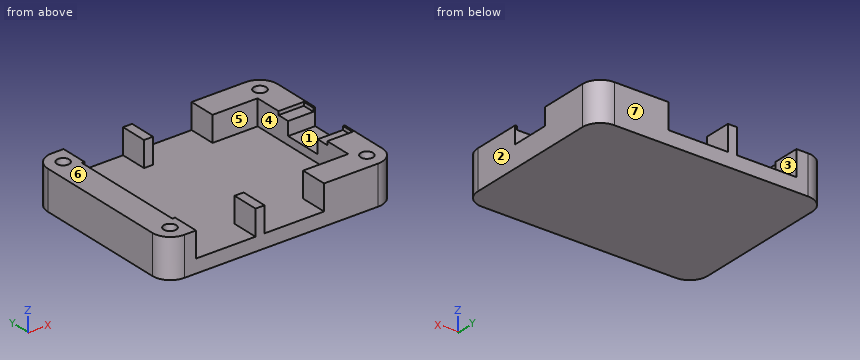
```python
from build123d import *

# Parameters (mm, degrees)
F0_R     = 2.6
F0_W     = 13.2
F0_H     = 6
F0_W_2   = 5.6
F0_H_2   = 8.5
F0_R_2   = 1.55
F0_H_3   = 2.75
F0_W_3   = 2
F0_R_3   = 1.375
F0_W_4   = 0.4
F1_DEPTH = 3
F2_DEPTH = 8.6
F3_DEPTH = 7.8
F4_DEPTH = 4.8


with BuildPart() as f1:
    # F0 (on Top) → F1 (new body)
    with BuildSketch(Plane.XY):
        Polygon((19.5, 13), (9.5, 13), (-3.7, 13), (-5.7, 13), (-18.9, 13), (-19.5, 13), (-19.5, -13), (-18.9, -13), (-5.7, -13), (-3.7, -13), (9.5, -13), (19.5, -13), (19.5, -7), (19.5, -4.25), (19.5, 4.25), (19.5, 7), align=None)
        with BuildLine():
            Line((-18.9, 13), (-18.9, 19))
            Line((-18.9, 19), (-21.5, 19))
            ThreePointArc((-21.5, 19), (-24.3284271247, 17.8284271247), (-25.5, 15))
            Line((-25.5, 15), (-25.5, -15))
            ThreePointArc((-25.5, -15), (-24.3284271247, -17.8284271247), (-21.5, -19))
            Line((-21.5, -19), (-18.9, -19))
            Line((-18.9, -19), (-18.9, -13))
            Line((-18.9, -13), (-19.5, -13))
            Line((-19.5, -13), (-19.5, 13))
            Line((-19.5, 13), (-18.9, 13))
        make_face()
        with Locations((-21.8334523779, -15.3334523779)):
            Circle(F0_R, mode=Mode.SUBTRACT)
        with Locations((-21.8334523779, 15.3334523779)):
            Circle(F0_R, mode=Mode.SUBTRACT)
        with BuildLine():
            Line((25.5, -15), (25.5, -7))
            Line((25.5, -7), (25.1, -7))
            Line((25.1, -7), (19.5, -7))
            Line((19.5, -7), (19.5, -13))
            Line((19.5, -13), (9.5, -13))
            Line((9.5, -13), (9.5, -19))
            Line((9.5, -19), (21.5, -19))
            ThreePointArc((21.5, -19), (24.3284271247, -17.8284271247), (25.5, -15))
        make_face()
        with Locations((21.8334523779, -15.3334523779)):
            Circle(F0_R, mode=Mode.SUBTRACT)
        with BuildLine():
            ThreePointArc((25.5, 15), (24.3284271247, 17.8284271247), (21.5, 19))
            Line((21.5, 19), (9.5, 19))
            Line((9.5, 19), (9.5, 13))
            Line((9.5, 13), (19.5, 13))
            Line((19.5, 13), (19.5, 7))
            Line((19.5, 7), (25.1, 7))
            Line((25.1, 7), (25.5, 7))
            Line((25.5, 7), (25.5, 15))
        make_face()
        with Locations((21.8334523779, 15.3334523779)):
            Circle(F0_R, mode=Mode.SUBTRACT)
        with Locations((-12.3, -16)):
            Rectangle(F0_W, F0_H)
        with Locations((2.9, 16)):
            Rectangle(F0_W, F0_H)
        with Locations((-12.3, 16)):
            Rectangle(F0_W, F0_H)
        with Locations((2.9, -16)):
            Rectangle(F0_W, F0_H)
        with Locations((22.3, 0)):
            Rectangle(F0_W_2, F0_H_2)
        with Locations((-21.8334523779, -15.3334523779)):
            Circle(F0_R)
        with Locations((-21.8334523779, -15.3334523779)):
            Circle(F0_R_2, mode=Mode.SUBTRACT)
        with Locations((21.8334523779, 15.3334523779)):
            Circle(F0_R)
        with Locations((21.8334523779, 15.3334523779)):
            Circle(F0_R_2, mode=Mode.SUBTRACT)
        with Locations((-21.8334523779, 15.3334523779)):
            Circle(F0_R)
        with Locations((-21.8334523779, 15.3334523779)):
            Circle(F0_R_2, mode=Mode.SUBTRACT)
        with Locations((21.8334523779, -15.3334523779)):
            Circle(F0_R)
        with Locations((21.8334523779, -15.3334523779)):
            Circle(F0_R_2, mode=Mode.SUBTRACT)
        with Locations((22.3, 5.625)):
            Rectangle(F0_W_2, F0_H_3)
        with Locations((22.3, -5.625)):
            Rectangle(F0_W_2, F0_H_3)
        with Locations((-4.7, -16)):
            Rectangle(F0_W_3, F0_H)
        with Locations((-4.7, 16)):
            Rectangle(F0_W_3, F0_H)
        with Locations((21.8334523779, 15.3334523779)):
            Circle(F0_R_2)
        with Locations((21.8334523779, 15.3334523779)):
            Circle(F0_R_3, mode=Mode.SUBTRACT)
        with Locations((-21.8334523779, -15.3334523779)):
            Circle(F0_R_2)
        with Locations((-21.8334523779, -15.3334523779)):
            Circle(F0_R_3, mode=Mode.SUBTRACT)
        with Locations((21.8334523779, -15.3334523779)):
            Circle(F0_R_2)
        with Locations((21.8334523779, -15.3334523779)):
            Circle(F0_R_3, mode=Mode.SUBTRACT)
        with Locations((-21.8334523779, 15.3334523779)):
            Circle(F0_R_2)
        with Locations((-21.8334523779, 15.3334523779)):
            Circle(F0_R_3, mode=Mode.SUBTRACT)
        with Locations((-21.8334523779, -15.3334523779)):
            Circle(F0_R_3)
        with Locations((-21.8334523779, 15.3334523779)):
            Circle(F0_R_3)
        with Locations((21.8334523779, -15.3334523779)):
            Circle(F0_R_3)
        with Locations((21.8334523779, 15.3334523779)):
            Circle(F0_R_3)
        with Locations((25.3, 0)):
            Rectangle(F0_W_4, F0_H_2)
        with Locations((25.3, 5.625)):
            Rectangle(F0_W_4, F0_H_3)
        with Locations((25.3, -5.625)):
            Rectangle(F0_W_4, F0_H_3)
    extrude(amount=F1_DEPTH)

    # F0 (on Top) → F2 (join)
    with BuildSketch(Plane.XY):
        with BuildLine():
            Line((-18.9, 13), (-18.9, 19))
            Line((-18.9, 19), (-21.5, 19))
            ThreePointArc((-21.5, 19), (-24.3284271247, 17.8284271247), (-25.5, 15))
            Line((-25.5, 15), (-25.5, -15))
            ThreePointArc((-25.5, -15), (-24.3284271247, -17.8284271247), (-21.5, -19))
            Line((-21.5, -19), (-18.9, -19))
            Line((-18.9, -19), (-18.9, -13))
            Line((-18.9, -13), (-19.5, -13))
            Line((-19.5, -13), (-19.5, 13))
            Line((-19.5, 13), (-18.9, 13))
        make_face()
        with Locations((-21.8334523779, -15.3334523779)):
            Circle(F0_R, mode=Mode.SUBTRACT)
        with Locations((-21.8334523779, 15.3334523779)):
            Circle(F0_R, mode=Mode.SUBTRACT)
        with BuildLine():
            ThreePointArc((25.5, 15), (24.3284271247, 17.8284271247), (21.5, 19))
            Line((21.5, 19), (9.5, 19))
            Line((9.5, 19), (9.5, 13))
            Line((9.5, 13), (19.5, 13))
            Line((19.5, 13), (19.5, 7))
            Line((19.5, 7), (25.1, 7))
            Line((25.1, 7), (25.5, 7))
            Line((25.5, 7), (25.5, 15))
        make_face()
        with Locations((21.8334523779, 15.3334523779)):
            Circle(F0_R, mode=Mode.SUBTRACT)
        with BuildLine():
            Line((25.5, -15), (25.5, -7))
            Line((25.5, -7), (25.1, -7))
            Line((25.1, -7), (19.5, -7))
            Line((19.5, -7), (19.5, -13))
            Line((19.5, -13), (9.5, -13))
            Line((9.5, -13), (9.5, -19))
            Line((9.5, -19), (21.5, -19))
            ThreePointArc((21.5, -19), (24.3284271247, -17.8284271247), (25.5, -15))
        make_face()
        with Locations((21.8334523779, -15.3334523779)):
            Circle(F0_R, mode=Mode.SUBTRACT)
        with Locations((21.8334523779, -15.3334523779)):
            Circle(F0_R)
        with Locations((21.8334523779, -15.3334523779)):
            Circle(F0_R_2, mode=Mode.SUBTRACT)
        with Locations((-21.8334523779, -15.3334523779)):
            Circle(F0_R)
        with Locations((-21.8334523779, -15.3334523779)):
            Circle(F0_R_2, mode=Mode.SUBTRACT)
        with Locations((-21.8334523779, 15.3334523779)):
            Circle(F0_R)
        with Locations((-21.8334523779, 15.3334523779)):
            Circle(F0_R_2, mode=Mode.SUBTRACT)
        with Locations((21.8334523779, 15.3334523779)):
            Circle(F0_R)
        with Locations((21.8334523779, 15.3334523779)):
            Circle(F0_R_2, mode=Mode.SUBTRACT)
        with Locations((-4.7, -16)):
            Rectangle(F0_W_3, F0_H)
        with Locations((-4.7, 16)):
            Rectangle(F0_W_3, F0_H)
        with Locations((21.8334523779, -15.3334523779)):
            Circle(F0_R_2)
        with Locations((21.8334523779, -15.3334523779)):
            Circle(F0_R_3, mode=Mode.SUBTRACT)
        with Locations((-21.8334523779, -15.3334523779)):
            Circle(F0_R_2)
        with Locations((-21.8334523779, -15.3334523779)):
            Circle(F0_R_3, mode=Mode.SUBTRACT)
        with Locations((-21.8334523779, 15.3334523779)):
            Circle(F0_R_2)
        with Locations((-21.8334523779, 15.3334523779)):
            Circle(F0_R_3, mode=Mode.SUBTRACT)
        with Locations((21.8334523779, 15.3334523779)):
            Circle(F0_R_2)
        with Locations((21.8334523779, 15.3334523779)):
            Circle(F0_R_3, mode=Mode.SUBTRACT)
        with Locations((25.3, 5.625)):
            Rectangle(F0_W_4, F0_H_3)
        with Locations((25.3, -5.625)):
            Rectangle(F0_W_4, F0_H_3)
    extrude(amount=F2_DEPTH)

    # F0 (on Top) → F3 (join)
    with BuildSketch(Plane.XY):
        with Locations((22.3, -5.625)):
            Rectangle(F0_W_2, F0_H_3)
        with Locations((22.3, 5.625)):
            Rectangle(F0_W_2, F0_H_3)
    extrude(amount=F3_DEPTH)

    # F0 (on Top) → F4 (join)
    with BuildSketch(Plane.XY):
        with Locations((22.3, 0)):
            Rectangle(F0_W_2, F0_H_2)
        with Locations((25.3, 0)):
            Rectangle(F0_W_4, F0_H_2)
    extrude(amount=F4_DEPTH)


solid = f1.part
```
Could you check a few things on this model? Use its own coordinates, in mm. Face numbers are marked on the shaded views. A direction names the side the tool comes from. Round coordinates to 2 decimals unless told otherwise and drop trailing zeros. Loops run counter-clockwise (first coordinate to the right, second up) from the corner with the lowest first, then second, coordinate; pieces in that order, holes last.
Q1. I want a section at A-A (y = -5). Write out the boundary of the cut face in (x, z).
Q2. I want a section at B-B (x = 16). Write out the boundary of the cut face in (y, z), and give its area (3 significant figures).
Q3. Please list where these lines run through material, in increasing order: L1, parallel to X at y = 5, z = 8; L2, parallel to Y at x = -5, z = 3.5; L3, parallel to X at y = 16, z = 6.5.
Q4. For P1, Ø3, axis at x = 22, y = -5, coming from the +Z side; P2, Ø5, axis at x = 23.5, y = 0.5, coming from the +Z side; P3, Ø4, axis at x = 16.5, y = 4, coming from the +Z side, each with a flat end and sliding along its axis, tell me the tip position at first contact or that it passes through.
Q5. Thinking about a two-plate mould opening in Y: for the marked faces 4, 5, 6 and 7, which applies, pulls with the +Y half, pulls with the -Y half, needs draft (parallel to the pull), parting line crosses it, or undercut?
Q6. I want a section at D-D (z = 6.5). Give the number of separate pieces and of enclosed holes in the cut face, and give its area (3 significant figures).
Q7. On a 3-axis mill with a long thin cutter (end or side, diameter ignored), from which of +Z, -Z, +X, -X, +Y, -Y can I reach the whole of each face in a straight line? I mean the marked faces 1, 2 and 3. Say none if no direction works.
Q8. I want a section at C-C (y = 8.5). Write out the boundary of the cut face in (x, z), and give its area (3 significant figures).
Answer below:
1. outline: (-25.5, 0) - (25.5, 0) - (25.5, 8.6) - (25.1, 8.6) - (25.1, 7.8) - (19.5, 7.8) - (19.5, 3) - (-19.5, 3) - (-19.5, 8.6) - (-25.5, 8.6) - close
2. outline: (-19, 0) - (19, 0) - (19, 8.6) - (13, 8.6) - (13, 3) - (-13, 3) - (-13, 8.6) - (-19, 8.6) - close
2. area: 181 mm2
3. L1: x = -25.5 to -19.5, 25.1 to 25.5
3. L2: y = -19 to -13, 13 to 19
3. L3: x = -25.37 to -23.04, -20.63 to -18.9, -5.7 to -3.7, 9.5 to 20.63, 23.04 to 25.37
4. P1: stops at z = 7.8
4. P2: stops at z = 4.8
4. P3: stops at z = 3
5. face 4: undercut
5. face 5: undercut
5. face 6: needs draft
5. face 7: pulls with the +Y half
6. separate pieces: 5
6. enclosed holes: 4
6. area: 519 mm2
7. face 1: +Z, +X
7. face 2: +Z, -Z, +X, +Y, -Y
7. face 3: +Z, +Y, -Y
8. outline: (-25.5, 0) - (25.5, 0) - (25.5, 8.6) - (19.5, 8.6) - (19.5, 3) - (-19.5, 3) - (-19.5, 8.6) - (-25.5, 8.6) - close
8. area: 220 mm2
